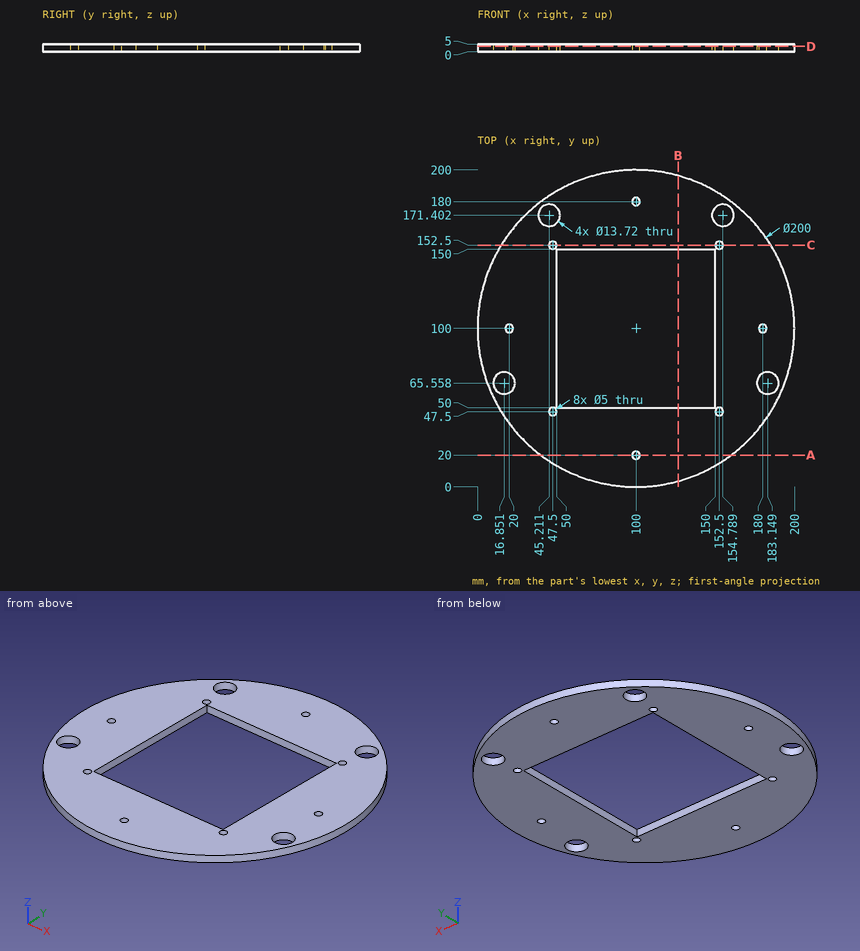
Here's the drawing with two shaded views (mm, measured from the low corner). I have some questions. Coordinates: 2 decimals unless noted, no trailing zeros. Order: outer loops, then holes, each group sorted by start corner. A loop starts at its lowest first (then second) coordinate and runs counter-clockwise, first axis right, second up.
Q1. Suppose I cut it at C-C on y = 152.5. Please give me the cut outline in (x, z).
Q2. Suppose I cut it at A-A on y = 20. Please give me the cut outline in (x, z).
Q3. Suppose I cut it at B-B on x = 126.5. Please give me the cut outline in (y, z) (1 decimal), and give its area (3 significant figures).
Q4. Please list where these lines run through material, in increasing order: L1, parallel to X at y = 152.5, z = 3.25; L2, parallel to X at y = 103, z = 2 (1 decimal); L3, parallel to Y at x = 47.5, z = 2.3 (1 decimal).
Q5. Suppose I cut it at D-D on z = 3.55. Give the number of separate pieces and of enclosed holes in the cut face, and give its area (3 significant figures).
Q6. Will these pins go through, and if not, where does the flat tip stop? pin 1 (11 mm diameter, centred on x = 154.79, y = 171.4, fed in from +Z); pin 2 (2 mm diameter, centred on y = 46.5, z = 4, fed in from +X); pin 3 (1 mm diameter, centred on y = 91, z = 0.5, fed in from +X); pin 4 (1.5 mm diameter, centred on y = 99, z = 1.5, fed in from +X).
Answer:
1. outline: (14.89, 0) - (45, 0) - (45, 5) - (14.89, 5) - close; (50, 0) - (150, 0) - (150, 5) - (50, 5) - close; (155, 0) - (185.11, 0) - (185.11, 5) - (155, 5) - close
2. outline: (40, 0) - (97.5, 0) - (97.5, 5) - (40, 5) - close; (102.5, 0) - (160, 0) - (160, 5) - (102.5, 5) - close
3. outline: (3.6, 0) - (50, 0) - (50, 5) - (3.6, 5) - close; (150, 0) - (196.4, 0) - (196.4, 5) - (150, 5) - close
3. area: 464 mm2
4. L1: x = 14.89 to 45, 50 to 150, 155 to 185.11
4. L2: x = 0 to 50, 150 to 200
4. L3: y = 14.9 to 45, 50 to 150, 155 to 164.9, 177.9 to 185.1
5. separate pieces: 1
5. enclosed holes: 13
5. area: 20,700 mm2
6. pin 1: passes through
6. pin 2: stops at x = 185.11
6. pin 3: stops at x = 199.64
6. pin 4: stops at x = 200
